Autodesk Inventor part; units mm, degrees
ref_plane "Start Plane" through (0, 0, 24.5) normal (0, 0, 1) x (1, 0, 0)
ref_plane "End Plane" through (0, 0, 290.1887) normal (0, 0, 1) x (1, 0, 0)
ref_plane "Work Plane4" through (12.7, 0, 290.1887) normal (0, 0.0180324, 0.9998374) x (1, 0, 0)
ref_plane "Start Plane" through (0, 0, 24.5) normal (0, 0, 1) x (1, 0, 0)
ref_plane "End Plane" through (0, 0, 290.1887) normal (0, 0, 1) x (1, 0, 0)
sketch "Sketch" plane through (0, 0, 0) normal (0, 0, 1) x (1, 0, 0)
  line L0 (25.4, 0) -> (0, 0)
  line L1 (0, 0) -> (0, 25.4)
  line L2 (0, 25.4) -> (1.651, 25.4)
  line L3 (3.175, 23.876) -> (3.175, 6.477)
  line L4 (6.477, 3.175) -> (23.876, 3.175)
  line L5 (25.4, 1.651) -> (25.4, 0)
  line L6 (0, -11.0414) -> (0, 31.5385) construction
  line L7 (-11.0414, 0) -> (31.5385, 0) construction
  arc A0 (3.175, 6.477) -> (6.477, 3.175) centre (6.477, 6.477) ccw
  arc A1 (3.175, 23.876) -> (1.651, 25.4) centre (1.651, 23.876) ccw
  arc A2 (25.4, 1.651) -> (23.876, 3.175) centre (23.876, 1.651) ccw
  line L8 (0, 40.0545) -> (0, -19.5574) construction
  line L9 (-19.5574, 0) -> (40.0545, 0) construction
  point P0 (3.175, 25.4)
  point P1 (3.175, 3.175)
  point P2 (25.4, 3.175)
  dimension "d0" = 25.4
  dimension "d1" = 25.4
  dimension "d2" = 3.175
  dimension "d3" = 3.175
  dimension "d10" = 0
  dimension "d11" = 0
  dimension "d14" = 3.302
  dimension "d15" = 1.524
extrude "Body" add sketch "Sketch" along normal up to surface (265.6887 mm away) from surface at 24.5
sketch "Sketch3" plane through (0, 0, 0) normal (0, 0, 1) x (1, 0, 0)
  line L0 (0, 0) -> (10, 0)
ref_plane "Work Plane3" through (0, 0, 0) normal (0, -1, 0) x (1, 0, 0)
ref_plane "Work Plane4" through (12.7, 0, 290.1887) normal (0, 0.0180324, 0.9998374) x (1, 0, 0)
split "Split1" plane through (12.7, 0, 290.1887) removes the side toward (0, 0.0180324, 0.9998374)
ref_plane "Work Plane9" through (690, 1039.3123, -12.0844) normal (0, -0.036059, -0.9993497) x (1, 0, 0)
split "Split3" plane through (690, 1039.3123, -12.0844) removes the side toward (0, -0.036059, -0.9993497)
sketch "Sketch4" plane through (0, 0, 0) normal (0, -1, 0) x (1, 0, 0)
  line L0 (-2, 24.5) -> (12, 24.5)
  line L1 (-2, 290.1887) -> (12, 290.1887)
  dimension "d17" = 265.6887
equation "\"d0\" = G_H"
equation "\"d1\" = G_H"
equation "\"d2\" = G_T"
equation "\"d3\" = G_T"
equation "\"d14\" = G_IR"
equation "\"d15\" = G_ER"
equation "\"d4\" = G_L"
equation "\"G_H\" = 25.4"
equation "\"G_T\" = 3.175"
equation "\"G_ER\" = 1.524"
equation "\"G_IR\" = 3.302"
equation "\"G_L\" = 265.68959"
equation "\"ex\" = 0"
equation "\"G_OFFSET_START\" = -24.50003"
equation "\"G_OFFSET_END\" = 0"
equation "\"d12\" = -G_OFFSET_START"
equation "\"d13\" = G_OFFSET_END + B_L"
equation "\"B_L\" = 290.18872"
properties part number "AISC - L 1 x 1 x 1/8 - 10.46" material "Steel, Mild"
Check sheet for the modelled part. Datum: model origin and axes. Units: mm. A direction names the side the tool comes from. Give positions to 0.01 mm unless a question says otherwise; leave off trailing zeros. Loops run counter-clockwise (first coordinate to the right, second up) from the corner with the lowest first, then second, coordinate; pieces in that order, holes last. Notation, with made-up numbers: M 34,52 L 42,52 A18 ccw 42,57 Z; hole C 61.5,26.5 d4. An arc over 180 degrees is marked long. Use a Markdown table: item, result. Add a question column.
Q1. Tool access check on faces 1 (the flat face through (0, 13, 155)), 2 (the flat face through (3.175, 15, 155)). Record the directions out of +Z, -Z, +X, -X, +Y, -Y that give a thin tool (end or side, any length) a straight path to the whole face; none if there is none.
Q2. Sectioned sample at A-A, the plane z = 108.5. Record the cut outline in (x, y) (3 decimals).
Q3. Sectioned sample at C-C, the plane y = 12.25. Record the cut outline in (x, z) (3 decimals), then the cut area to 3 significant figures.
Q4. Go/stop test with flat-tipped pins: pin 1 (5 mm diameter, centred on y = 12, z = 99.5, fed in from -X); pin 2 (8 mm diameter, centred on y = 21, z = 247.5, fed in from +X) (3 decimals). Record where each tip stops, or that it passes through.
Q5. Scan lines: line 1 along X through (y, z) = (18, 134) (3 decimals); line 2 along Z through (x, y) = (17.25, 2). Record each from-to range of solid material in increasing order. Write a range as [from, to].
Q6. Sectioned sample at B-B, the plane x = 14.25. Record the cut outline in (y, z) (3 decimals).
Verdict:
| question | item | result |
|---|---|---|
| 1 | face 1 | +Z, -Z, -X, +Y, -Y |
| 1 | face 2 | +Z, -Z, +X, +Y |
| 2 | outline | M 0,0 L 25.4,0 L 25.4,1.651 A1.524 ccw 23.876,3.175 L 6.477,3.175 A3.302 cw 3.175,6.477 L 3.175,23.876 A1.524 ccw 1.651,25.4 L 0,25.4 Z |
| 3 | outline | M 0,24.975 L 3.175,24.975 L 3.175,289.968 L 0,289.968 Z |
| 3 | area | 841 mm^2 |
| 4 | pin 1 | x = 0 |
| 4 | pin 2 | x = 3.175 |
| 5 | line 1 | [0, 3.175] |
| 5 | line 2 | [25.34, 290.15] |
| 6 | outline | M 0,25.417 L 3.175,25.302 L 3.175,290.131 L 0,290.189 Z |
